For this review, take the finished solid that the model builds, in its own axes (mm). Face numbers are marked on the shaded views. Coordinates: 2 decimals unless noted, no trailing zeros. Order: outer loops, then holes, each group sorted by start corner. A loop starts at its lowest first (then second) coordinate and runs counter-clockwise, first axis right, second up. Notation, with made-up numbers: M 39.5,60 L 55.5,60 A28 cw 55.5,99 Z; hole C -34.75,76.5 d8. An arc over 180 degrees is marked long. Use CSV: the item, a comma, the result in double quotes.
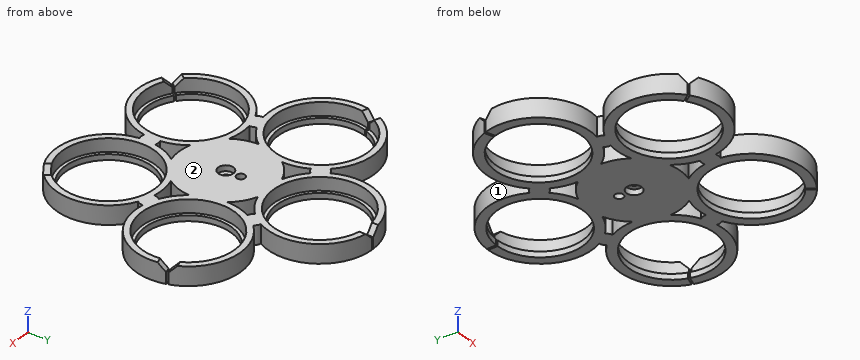
Autodesk Inventor part; units mm, degrees
ref_plane "YZ Plane" through (0, 0, 0) normal (1, 0, 0) x (0, 1, 0)
ref_plane "XZ Plane" through (0, 0, 0) normal (0, 1, 0) x (-1, 0, 0)
ref_plane "XY Plane" through (0, 0, 0) normal (0, 0, 1) x (1, 0, 0)
sketch "Sketch1" plane through (0, 0, 0) normal (0, 0, 1) x (1, 0, 0)
  arc A0 (-0.4512, 77.997) -> (0.5077, 77.9956) centre (-0.0102, 50) ccw
  arc A1 (-0.4697, 74.7457) -> (0.4892, 74.745) centre (-0.0102, 50) ccw
  arc A2 (-0.4796, 72.9952) -> (0.4793, 72.9948) centre (-0.0102, 50) ccw
  line L0 (0.5077, 77.9956) -> (0.4793, 72.9948)
  line L1 (-0.4697, 74.7457) -> (-0.4512, 77.997)
  line L2 (-0.4796, 72.9952) -> (-0.4697, 74.7457)
  arc A3 (-74.3189, 23.6733) -> (-74.0214, 24.5848) centre (-47.556, 15.4411) ccw
  arc A4 (-71.2326, 22.651) -> (-70.9355, 23.5627) centre (-47.556, 15.4411) ccw
  arc A5 (-69.5708, 22.1006) -> (-69.2741, 23.0125) centre (-47.556, 15.4411) ccw
  line L3 (-74.0214, 24.5848) -> (-69.2741, 23.0125)
  line L4 (-71.2326, 22.651) -> (-74.3189, 23.6733)
  line L5 (-69.5708, 22.1006) -> (-71.2326, 22.651)
  arc A6 (-45.4804, -63.3661) -> (-46.2554, -62.8014) centre (-29.381, -40.4568) ccw
  arc A7 (-43.5545, -60.7466) -> (-44.3298, -60.1824) centre (-29.381, -40.4568) ccw
  arc A8 (-42.5175, -59.3363) -> (-43.293, -58.7723) centre (-29.381, -40.4568) ccw
  line L6 (-46.2554, -62.8014) -> (-43.293, -58.7723)
  line L7 (-43.5545, -60.7466) -> (-45.4804, -63.3661)
  line L8 (-42.5175, -59.3363) -> (-43.5545, -60.7466)
  arc A9 (46.2105, -62.8357) -> (45.434, -63.3982) centre (29.3975, -40.4449) ccw
  arc A10 (44.3144, -60.1945) -> (43.5382, -60.7575) centre (29.3975, -40.4449) ccw
  arc A11 (43.2935, -58.7725) -> (42.5175, -59.3357) centre (29.3975, -40.4449) ccw
  line L9 (45.434, -63.3982) -> (42.5175, -59.3357)
  line L10 (44.3144, -60.1945) -> (46.2105, -62.8357)
  line L11 (43.2935, -58.7725) -> (44.3144, -60.1945)
  arc A12 (74.0401, 24.5315) -> (74.3351, 23.6192) centre (47.5497, 15.4606) ccw
  arc A13 (70.9423, 23.5444) -> (71.2379, 22.6322) centre (47.5497, 15.4606) ccw
  arc A14 (69.2744, 23.0129) -> (69.5703, 22.1008) centre (47.5497, 15.4606) ccw
  line L12 (74.3351, 23.6192) -> (69.5703, 22.1008)
  line L13 (70.9423, 23.5444) -> (74.0401, 24.5315)
  line L14 (69.2744, 23.0129) -> (70.9423, 23.5444)
  circle A15 centre (0, 0) radius 24.9
  circle A16 centre (0, 0) radius 1.5
  circle A17 centre (0, 8) radius 1.25
  circle A18 centre (0, -40.4449) radius 4.5
  circle A19 centre (38.4653, -12.4981) radius 4.5
  circle A20 centre (23.7729, 32.7206) radius 4.5
  circle A21 centre (-23.7729, 32.7206) radius 4.5
  circle A22 centre (-38.4653, -12.4981) radius 4.5
  point P0 (0, 77.029)
  point P1 (-73.2589, 23.8033)
  point P2 (-45.2765, -62.3177)
  point P3 (45.2765, -62.3177)
  point P4 (73.2589, 23.8033)
  dimension "d5" = 50
  dimension "d8" = 360
  dimension "d10" = 3
  dimension "d11" = 2.5
  dimension "d14" = 24.75
  dimension "d20" = 9
  dimension "d21" = 23
  dimension "d24" = 360
extrude "Extrusion1" add sketch "Sketch1" along normal blind 10 contours L1 A1 L0 A0 A20 A15 A21 | A21 A0 | A21 A3 A15 A22 L4 A4 L3 | A3 A21 | A15 A0 | A0 A15 A12 A9 A6 A3 | A3 A15 | A0 A20 | A15 A12 | A12 A20 L13 A13 L12 A19 A15 | A20 A12 | A3 A22 | A15 A6 A18 L7 A7 L6 A22 | A6 A15 | A19 A12 | A15 A9 | A9 A19 L10 A10 L9 A18 A15 | A22 A6 | A9 A19 | A6 A18 | A18 A9
sketch "Sketch2" plane through (0, 0, 10) normal (0, 0, 1) x (1, 0, 0)
  circle A0 centre (0, 0) radius 4.05
  circle A1 centre (0, 8) radius 1.25
  circle A2 centre (0, 8) radius 2.25
  dimension "d15" = 8.1
  dimension "d35" = 4.5
extrude "Extrusion2" cut sketch "Sketch2" against normal blind 3 contours A0
extrude "Extrusion3" add sketch "Sketch1" along normal blind 3 contours L2 A2 L0 A1 | A4 L5 A5 L3 | L14 A14 L12 A13 | A7 L8 A8 L6 | L11 A11 L9 A10
extrude "Extrusion4" add sketch "Sketch1" along normal blind 10 contours A21 A0 | A0 A21 A3 | A3 A21 | A20 A12 A0 | A0 A20 | A20 A12 | A22 A6 A3 | A3 A22 | A19 A12 | A12 A19 A9 | A22 A6 | A9 A19 | A18 A9 A6 | A6 A18 | A18 A9
sketch "Sketch3" plane through (0, 0, 0) normal (0, 0, -1) x (-1, 0, 0)
  circle A0 centre (0, 0) radius 1.5
  circle A1 centre (0, 0) radius 4.05
  circle A2 centre (0, 8) radius 1.25
  circle A3 centre (0, 8) radius 2.25
  dimension "d28" = 8.1
  dimension "d29" = 4.5
extrude "Extrusion5" cut sketch "Sketch3" against normal blind 3
chamfer "Chamfer1" distance 4 angle 45 10 edges at (-72.4784, 24.0738, 10) (-72.7758, 23.1621, 10) (-0.4604, 76.3713, 10) (0.4984, 76.3703, 10) (72.4912, 24.0379, 10) (72.7865, 23.1257, 10) (45.2625, -61.5151, 10) (44.4861, -62.0779, 10) (-45.2926, -61.4919, 10) (-44.5175, -62.0564, 10)
extrude "Extrusion6" cut sketch "Sketch2" against normal blind 3 contours A2
properties part number "FilterWheel-2inch-5pos"
Item 1: Draft analysis for pull direction Y (two halves, no side actions). For the marked faces 1 and 2, state which applies: released by +Y, released by -Y, zero draft, split by the parting line, or undercut.
Solutions:
face 1,"undercut"
face 2,"zero draft"
Item 2: Add section A-A on y = -42.5. State the section outline as (x, z) points, and give its area (3 significant figures).
Solutions:
outline,"M -57.31,0 L -52.29,0 L -52.29,3 L -54.05,3 L -54.05,10 L -57.31,10 Z; M -6.47,0 L 6.49,0 L 6.49,3 L 4.73,3 L 4.73,10 L -4.72,10 L -4.72,3 L -6.47,3 Z; M 52.31,0 L 57.32,0 L 57.32,10 L 54.06,10 L 54.06,3 L 52.31,3 Z"
area,"181 mm^2"
Item 3: To check wall thickness, follow line 1 along Y through (x, z) = (0, 5.85); line 2 along X through (y, z) = (0, 3.25); line 3 along X through (y, z) = (-25, 1.5). State the ranges of each line that lie inside material, in increasing order. Write a range as [from, to].
Solutions:
line 1,"[-44.94, -35.94], [-24.9, -1.5], [1.5, 6.75], [9.25, 25.25]"
line 2,"[-70.91, -66.9], [-28.21, -1.5], [1.5, 28.22], [66.88, 70.89]"
line 3,"[-52.73, -46.41], [-12.35, -6.03], [6.04, 12.36], [46.44, 52.75]"
Item 4: Add section B-B on x = 31.5. State the section outline as (y, z) points.
Solutions:
outline,"M -68.37,0 L -63.35,0 L -63.35,3 L -65.11,3 L -65.11,10 L -68.37,10 Z; M -17.54,0 L -12.52,0 L -12.52,10 L -15.78,10 L -15.78,3 L -17.54,3 Z; M -7.48,0 L -1.01,0 L -1.01,3 L -3.38,3 L -3.38,10 L -7.48,10 Z; M 31.94,0 L 38.41,0 L 38.41,10 L 34.3,10 L 34.3,3 L 31.94,3 Z"
Item 5: Clearance check with flat-ended pins moving along their axes: pin 1 Ø1.5 at (x, z) = (-34.5, 7.5) entering from -Y; pin 2 Ø4 at (x, y) = (0, 8) entering from +Z; pin 3 Ø4 at (y, z) = (-6.5, 5) entering from -X; pin 4 Ø13 at (x, y) = (0, 0) entering from -Z. State where each tip first meets the part, or that it passes through.
Solutions:
pin 1,"y = -68.11"
pin 2,"z = 7"
pin 3,"x = -67.21"
pin 4,"z = 0"
Item 6: Add section C-C on y = 63.5. State the section outline as (x, z) points.
Solutions:
outline,"M -24.54,0 L -18.63,0 L -18.63,3 L -20.75,3 L -20.75,10 L -24.54,10 Z; M 18.61,0 L 24.52,0 L 24.52,10 L 20.74,10 L 20.74,3 L 18.61,3 Z"
Item 7: Add section D-D on y = -27. State the section outline as (x, z) points, and give its area (3 significant figures).
Solutions:
outline,"M -53.94,0 L -48.03,0 L -48.03,3 L -50.15,3 L -50.15,10 L -53.94,10 Z; M -10.73,0 L -4.83,0 L -4.83,10 L -8.61,10 L -8.61,3 L -10.73,3 Z; M 4.84,0 L 10.74,0 L 10.74,3 L 8.62,3 L 8.62,10 L 4.84,10 Z; M 48.06,0 L 53.96,0 L 53.96,10 L 50.18,10 L 50.18,3 L 48.06,3 Z"
area,"177 mm^2"
